Here's how the part is built. I have some questions about the finished solid (model axes, mm). Coordinates: 2 decimals unless noted, no trailing zeros. Loops run counter-clockwise (first coordinate to the right, second up) from the corner with the lowest first, then second, coordinate; pieces in that order, holes last. Notation, with made-up numbers: (-30.75, -32) -> (-12.75, -32) arc R22 ccw to (-12.75, 7) -> close; hole circle Ø3 at (16.25, 1.5). An arc over 180 degrees is marked (long way). Answer as a JSON object with one key per item and string values. Group by question number.
Q1. I want a section at D-D on z = 9.75. Write out the boundary of the cut face in (x, y), then the cut area to 3 significant figures.
Q2. I want a section at A-A on y = 0.65. Write out the boundary of the cut face in (x, z).
Q3. I want a section at B-B on z = 5.5. Write out the boundary of the cut face in (x, y).
Q4. I need wall thicknesses on line 1 (Y direction, x = 0.95, z = 5); line 2 (Z direction, x = 0.55, y = 0.65); line 3 (Z direction, x = 0.5, y = 1.5). Which ranges of each line are inside material? Lowest first, please.
Q5. Thinking about a two-plate mould opening in Y: for faces 1 (the cylindrical face through (-1.05, 3.92, 4.93)), 2 (the flat face through (0, 0, 10)), 3 (the cylindrical face through (0.02, -0.4, 2.46)), 4 (the flat face through (0, -4.35, 5)), which applies, released by +Y, released by -Y, zero draft, split by the parting line, or undercut?
Q6. I want a section at C-C on x = -1.15. Write out the boundary of the cut face in (y, z), then the cut area to 3 significant figures.
```python
from build123d import *

# Parameters (mm, degrees)
SKETCH_1_W          = 3
SKETCH_1_H          = 8.7
EXTRUDE_1_DEPTH     = 10
SKETCH_2_R          = 2.75
CUT_EXTRUDE_1_DEPTH = 10
FILLET_1_R          = 1.5


with BuildPart() as part:
    # 草图1 → 凸台-拉伸1 (new body)
    with BuildSketch(Plane.XY):
        Rectangle(SKETCH_1_W, SKETCH_1_H)
    extrude(amount=EXTRUDE_1_DEPTH)

    # 草图2 → 切除-拉伸1 (cut)
    with BuildSketch(Plane(origin=(1.5, 0, 0), x_dir=(0, 0, -1), z_dir=(1, 0, 0))):
        with Locations((-5, 0.65)):
            Circle(SKETCH_2_R)
    extrude(amount=-CUT_EXTRUDE_1_DEPTH, mode=Mode.SUBTRACT)

    # 圆角1
    # the kernel refuses this fillet: 1.5 mm, written as the material it takes off along each edge
    with BuildSketch(Plane(origin=(-1.5, 4.35, -3.75), x_dir=(0, -1, 0), z_dir=(0, 0, 1))) as fillet_1_piece_1:
        with BuildLine():
            CenterArc((FILLET_1_R, FILLET_1_R), FILLET_1_R, 180, 90)
            Line((0, FILLET_1_R), (0, 0))
            Line((0, 0), (FILLET_1_R, 0))
        make_face()
    extrude(amount=17.5, mode=Mode.SUBTRACT)


solid = part.part
```
Result set:
{
 "1": {"outline": "(-1.5, -4.35) -> (1.5, -4.35) -> (1.5, 4.35) -> (0, 4.35) arc R1.5 ccw to (-1.5, 2.85) -> close", "area": "25.6 mm²"},
 "2": {"outline": "(-1.5, 0) -> (1.5, 0) -> (1.5, 2.25) -> (-1.5, 2.25) -> close; (-1.5, 7.75) -> (1.5, 7.75) -> (1.5, 10) -> (-1.5, 10) -> close"},
 "3": {"outline": "(-1.5, -4.35) -> (1.5, -4.35) -> (1.5, -2.05) -> (-1.5, -2.05) -> close; (-1.41, 3.35) -> (1.5, 3.35) -> (1.5, 4.35) -> (0, 4.35) arc R1.5 ccw to start"},
 "4": {"line 1": "y = -4.35 to -2.1, 3.4 to 4.35", "line 2": "z = 0 to 2.25, 7.75 to 10", "line 3": "z = 0 to 2.38, 7.62 to 10"},
 "5": {"face 1": "released by +Y", "face 2": "zero draft", "face 3": "undercut", "face 4": "released by -Y"},
 "6": {"outline": "(-4.35, 0) -> (3.81, 0) -> (3.81, 10) -> (-4.35, 10) -> close; hole circle Ø5.5 at (0.65, 5)", "area": "57.9 mm²"}
}
